Geometry: final body of the model. Coordinates: model frame, mm. A direction names the side the tool comes from. Give positions to 0.01 mm unless a question says otherwise; leave off trailing zeros. Order: outer loops, then holes, each group sorted by start corner. A loop starts at its lowest first (then second) coordinate and runs counter-clockwise, first axis right, second up. Notation, with made-up numbers: (54, 53.25) - (80, 53.25) arc R15 ccw to (80, 60.25) - close; hole circle Ø10 at (1.5, -13). An arc over 180 degrees is marked (long way). Use one line per item in the form item = value.
from build123d import *

# Parameters (mm, degrees)
SKETCH_HOUSING_PROFILE_W             = 50
SKETCH_HOUSING_PROFILE_H             = 35
HOUSING_BLOCK_72X50X35_DEPTH         = 72
SKETCH_WEB_CLEARANCE_HOLE_9_R        = 4.5
WEB_CLEARANCE_HOLE_9_DEPTH           = 3
SKETCH_REAR_BUSHING_BORE_12_R        = 6
REAR_BUSHING_BORE_12_H7_DEPTH        = 12
SKETCH_SPRING_BORE_13_R              = 6.5
SPRING_POCKET_BORE_13_DEPTH          = 40
SKETCH_FRONT_BUSHING_BORE_18_R       = 9
FRONT_BUSHING_BORE_18_H7_DEPTH       = 17
SKETCH_MOUNTING_CLEARANCE_HOLES_M5_R = 2.75
MOUNTING_CLEARANCE_HOLES_M5_DEPTH    = 35
SKETCH_MOUNTING_COUNTERBORES_9_R     = 4.5
MOUNTING_COUNTERBORES_9X5P4_DEPTH    = 5.4


with BuildPart() as part:
    # Sketch_Housing_Profile → Housing_Block_72x50x35 (new body)
    with BuildSketch(Plane(origin=(0, 0, 0), x_dir=(0, 0, -1), z_dir=(1, 0, 0))):
        with Locations((0, -2.5)):
            Rectangle(SKETCH_HOUSING_PROFILE_W, SKETCH_HOUSING_PROFILE_H)
    extrude(amount=HOUSING_BLOCK_72X50X35_DEPTH)

    # Sketch_Web_Clearance_Hole_9 → Web_Clearance_Hole_9 (cut)
    with BuildSketch(Plane(origin=(0, 0, 0), x_dir=(0, 0, -1), z_dir=(1, 0, 0))):
        Circle(SKETCH_WEB_CLEARANCE_HOLE_9_R)
    extrude(amount=WEB_CLEARANCE_HOLE_9_DEPTH, mode=Mode.SUBTRACT)

    # Sketch_Rear_Bushing_Bore_12 → Rear_Bushing_Bore_12_H7 (cut)
    with BuildSketch(Plane(origin=(3, 0, 0), x_dir=(0, 0, -1), z_dir=(1, 0, 0))):
        Circle(SKETCH_REAR_BUSHING_BORE_12_R)
    extrude(amount=REAR_BUSHING_BORE_12_H7_DEPTH, mode=Mode.SUBTRACT)

    # Sketch_Spring_Bore_13 → Spring_Pocket_Bore_13 (cut)
    with BuildSketch(Plane(origin=(15, 0, 0), x_dir=(0, 0, -1), z_dir=(1, 0, 0))):
        Circle(SKETCH_SPRING_BORE_13_R)
    extrude(amount=SPRING_POCKET_BORE_13_DEPTH, mode=Mode.SUBTRACT)

    # Sketch_Front_Bushing_Bore_18 → Front_Bushing_Bore_18_H7 (cut)
    with BuildSketch(Plane(origin=(55, 0, 0), x_dir=(0, 0, -1), z_dir=(1, 0, 0))):
        Circle(SKETCH_FRONT_BUSHING_BORE_18_R)
    extrude(amount=FRONT_BUSHING_BORE_18_H7_DEPTH, mode=Mode.SUBTRACT)

    # Sketch_Mounting_Clearance_Holes_M5 → Mounting_Clearance_Holes_M5 (cut)
    with BuildSketch(Plane(origin=(0, 15, 0), x_dir=(1, 0, 0), z_dir=(0, 1, 0))):
        with Locations(Location((11, 17, 0), (0, 0, 270))):
            Circle(SKETCH_MOUNTING_CLEARANCE_HOLES_M5_R)
        with Locations(Location((61, 17, 0), (0, 0, 270))):
            Circle(SKETCH_MOUNTING_CLEARANCE_HOLES_M5_R)
        with Locations(Location((11, -17, 0), (0, 0, 270))):
            Circle(SKETCH_MOUNTING_CLEARANCE_HOLES_M5_R)
        with Locations(Location((61, -17, 0), (0, 0, 270))):
            Circle(SKETCH_MOUNTING_CLEARANCE_HOLES_M5_R)
    extrude(amount=-MOUNTING_CLEARANCE_HOLES_M5_DEPTH, mode=Mode.SUBTRACT)

    # Sketch_Mounting_Counterbores_9 → Mounting_Counterbores_9x5p4 (cut)
    with BuildSketch(Plane(origin=(0, 15, 0), x_dir=(1, 0, 0), z_dir=(0, 1, 0))):
        with Locations(Location((11, 17, 0), (0, 0, 270))):
            Circle(SKETCH_MOUNTING_COUNTERBORES_9_R)
        with Locations(Location((61, 17, 0), (0, 0, 270))):
            Circle(SKETCH_MOUNTING_COUNTERBORES_9_R)
        with Locations(Location((11, -17, 0), (0, 0, 270))):
            Circle(SKETCH_MOUNTING_COUNTERBORES_9_R)
        with Locations(Location((61, -17, 0), (0, 0, 270))):
            Circle(SKETCH_MOUNTING_COUNTERBORES_9_R)
    extrude(amount=-MOUNTING_COUNTERBORES_9X5P4_DEPTH, mode=Mode.SUBTRACT)


solid = part.part
(1) Reachability of faces 5 (the face through (15, -6, -2)), 6 (the face through (11.198, 12.338, -21.496)), 7 (the face through (1.48, 4.46, 0.59)) from +Z, -Z, +X, -X, +Y, -Y: full face, straight path, thin tool, end or side. Return the list, or none.
Computed values:
face_5 = +X
face_6 = +Y
face_7 = +X, -X
(2) Cut plane C-C on z = 0. Output: boundary loops of the cut face in (x, y), plus the area to 3 significant figures.
Computed values:
outline = (0, -20) - (72, -20) - (72, -9) - (55, -9) - (55, -6.5) - (15, -6.5) - (15, -6) - (3, -6) - (3, -4.5) - (0, -4.5) - close; (0, 4.5) - (3, 4.5) - (3, 6) - (15, 6) - (15, 6.5) - (55, 6.5) - (55, 9) - (72, 9) - (72, 15) - (0, 15) - close
area = 1,520 mm²
(3) Cut plane D-D on y = 12.5. Output: boundary loops of the cut face in (x, z).
Computed values:
outline = (0, -25) - (72, -25) - (72, 25) - (0, 25) - close; hole circle Ø9 at (11, -17); hole circle Ø9 at (11, 17); hole circle Ø9 at (61, -17); hole circle Ø9 at (61, 17)
(4) Pull-direction query (Y, two-part tool) for faces 1 (the face through (12.859, -4.993, -19.027)), 2 (the face through (34.72, -3.955, 5.158)), 3 (the face through (63.381, 8.923, 1.172)), 4 (the face through (35, -20, 0)); classes: released by +Y, released by -Y, zero draft, split by the parting line, or undercut.
Computed values:
face_1 = zero draft
face_2 = undercut
face_3 = undercut
face_4 = released by -Y
(5) Cut plane B-B on x = 61. Output: boundary loops of the cut face in (y, z), plus the area to 3 significant figures.
Computed values:
outline = (-20, -25) - (15, -25) - (15, -21.5) - (9.6, -21.5) - (9.6, -19.75) - (-20, -19.75) - close; (-20, -14.25) - (9.6, -14.25) - (9.6, -12.5) - (15, -12.5) - (15, 12.5) - (9.6, 12.5) - (9.6, 14.25) - (-20, 14.25) - close; (-20, 19.75) - (9.6, 19.75) - (9.6, 21.5) - (15, 21.5) - (15, 25) - (-20, 25) - close; hole circle Ø18 at (0, 0)
area = 1,070 mm²
(6) Cut plane A-A on y = 0. Output: boundary loops of the cut face in (x, z).
Computed values:
outline = (0, -25) - (72, -25) - (72, -9) - (55, -9) - (55, -6.5) - (15, -6.5) - (15, -6) - (3, -6) - (3, -4.5) - (0, -4.5) - close; (0, 4.5) - (3, 4.5) - (3, 6) - (15, 6) - (15, 6.5) - (55, 6.5) - (55, 9) - (72, 9) - (72, 25) - (0, 25) - close; hole circle Ø5.5 at (11, -17); hole circle Ø5.5 at (11, 17); hole circle Ø5.5 at (61, -17); hole circle Ø5.5 at (61, 17)
(7) Ray query, line 1 along X through (y, z) = (1.5, 17); line 2 along X through (y, z) = (13.8, -17); line 3 along Y through (x, z) = (23, 0). Return the intervals inside material, ascending.
Computed values:
line_1 = 0 to 8.25, 13.75 to 58.25, 63.75 to 72
line_2 = 0 to 6.5, 15.5 to 56.5, 65.5 to 72
line_3 = -20 to -6.5, 6.5 to 15
(8) Contact query for flat-ended pins moving along their axis: pin 1 Ø7 at (x, z) = (11, -17) entering from +Y; pin 2 Ø10.5 at (y, z) = (0, 0) entering from +X; pin 3 Ø15 at (y, z) = (0, 0) entering from +X. Output: stop coordinate, or through.
Computed values:
pin_1 = 9.6
pin_2 = 3
pin_3 = 55
